Build history of the part. All positions in model axes, mm. Face numbers are marked on the shaded views. A direction names the side the tool comes from. Round coordinates to 2 decimals unless told otherwise and drop trailing zeros. Order: outer loops, then holes, each group sorted by start corner. A loop starts at its lowest first (then second) coordinate and runs counter-clockwise, first axis right, second up. Notation, with made-up numbers: M -31.75,81.5 L 26.25,81.5 A11 ccw 26.25,100.5 Z; hole C 18.25,81.25 d8. An arc over 180 degrees is marked long. One line per item, written item: value. Start each with the question number.
Item 1: Pin check, flat tips, straight feed: pin 1 (3 mm diameter, centred on y = 0.5, z = -3.5, fed in from -X); pin 2 (3 mm diameter, centred on x = -11, y = 1.5, fed in from -Z); pin 3 (2 mm diameter, centred on x = -12, z = 5, fed in from -Y). Stop position of each tip, or through.
Item 2: Tool access for the marked faces 4, 5, 6 and 7: list every direction of +Z, -Z, +X, -X, +Y, -Y with a clear straight run to the whole face (end or side of a thin tool).
Item 3: Band-saw the part on C-C, the plane y = 3.75. Write the cut outline in (x, z).
Item 4: Two-plate mould, pull along Y, no slides. Class the marked faces 1, 2 and 3: +Y half, -Y half, draft (parallel to the pull), parting line (faces both ways), or undercut.
Item 5: Band-saw the part on B-B, the plane z = 2.25. Give the number of separate pieces and of enclosed holes in the cut face, then the cut area to 3 significant figures.
Item 6: Probe L1, parallel to X at y = -3, z = 0.25; L2, parallel to X at y = -1.5, z = 5; L3, parallel to X at y = -4, z = 5.75. List the from-to ranges inside material, lowest first.
Item 7: Band-saw the part on A-A, the plane z = -2.25. Write the cut outline in (x, y), then the cut area to 3 significant figures.
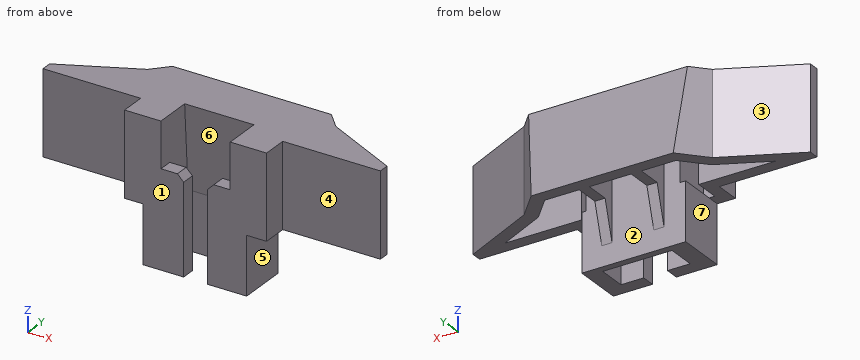
```python
from build123d import *

# Parameters (mm, degrees)
BOSS_EXTRUDE1_DEPTH = 7.4
CUT_EXTRUDE1_DEPTH  = 31.916943618
CHAMFER1_SIZE       = 0.5
CHAMFER1_SIZE_2     = 8
BOSS_EXTRUDE2_DEPTH = 5.1
SKETCH8_W           = 2
SKETCH8_H           = 3.4
BOSS_EXTRUDE5_DEPTH = 1.2
CHAMFER2_SIZE       = 0.55
BOSS_EXTRUDE6_REACH = 19.155
SKETCH9_W           = 0.9
SKETCH9_H           = 3.093590623
SKETCH10_W          = 0.9
SKETCH10_H          = 3.309924143
BOSS_EXTRUDE7_DEPTH = 1
CHAMFER3_SIZE       = 3.5
CHAMFER3_SIZE_2     = 1


with BuildPart() as part:
    # Sketch1 → Boss-Extrude1 (new body)
    with BuildSketch(Plane.XY):
        Polygon((-6.25, 4.137675877), (6.25, 4.137675877), (8.287698915, 1.935907694), (14.849810865, -1.262324123), (14.849810865, -2.162324123), (6.250723489, -2.162324123), (6.25, -4.362324123), (3.05, -4.362324123), (3.05, -1.162324123), (-3.05, -1.162324123), (-3.05, -4.362324123), (-6.25, -4.362324123), (-6.25, -2.162324123), (-14.849810865, -2.162324123), (-14.849810865, -1.262324123), (-8.287698915, 1.935907694), align=None)
    extrude(amount=BOSS_EXTRUDE1_DEPTH)

    # Sketch3 → Cut-Extrude1 (cut, through all)
    with BuildSketch(Plane(origin=(14.849810865, 0, 0), x_dir=(0, 0, -1), z_dir=(1, 0, 0))):
        Polygon((-7.4, 3.337675877), (0, 4.137675877), (-7.4, 4.137675877), align=None)
    extrude(amount=-CUT_EXTRUDE1_DEPTH, mode=Mode.SUBTRACT)

    # Shell1: read off the stored shape, not the designer's step
    # Shell1: loft between two sections, ruled curve by curve
    shell1_from = [
        Edge.make_line((5.15, -1.062324123, 6.3), (11.928689782, -1.062324123, 6.3)),
        Edge.make_line((-11.928689782, -1.062324123, 6.3), (-5.15, -1.062324123, 6.3)),
        Edge.make_line((11.928689782, -1.062324123, 6.3), (7.620430834, 1.037428357, 6.3)),
        Edge.make_line((7.620430834, 1.037428357, 6.3), (6.405496555, 2.350185419, 6.3)),
        Edge.make_line((-6.405496555, 2.350185419, 6.3), (-7.620430834, 1.037428357, 6.3)),
        Edge.make_line((-7.620430834, 1.037428357, 6.3), (-11.928689782, -1.062324123, 6.3)),
        Edge.make_line((-5.15, -1.062324123, 6.3), (-5.15, -3.262324123, 6.3)),
        Edge.make_line((-5.15, -3.262324123, 6.3), (-4.15, -3.262324123, 6.3)),
        Edge.make_line((4.15, -3.262324123, 6.3), (5.15, -3.262324123, 6.3)),
        Edge.make_line((-4.15, -3.262324123, 6.3), (-4.15, -0.062324123, 6.3)),
        Edge.make_line((-4.15, -0.062324123, 6.3), (4.15, -0.062324123, 6.3)),
        Edge.make_line((4.15, -0.062324123, 6.3), (4.15, -3.262324123, 6.3)),
        Edge.make_line((5.15, -3.262324123, 6.3), (5.15, -1.062324123, 6.3)),
        Edge.make_line((6.405496555, 2.350185419, 6.3), (-6.405496555, 2.350185419, 6.3)),
    ]
    shell1_to = [
        Edge.make_line((5.15, -1.062324123, 0), (11.928689782, -1.062324123, 0)),
        Edge.make_line((-11.928689782, -1.062324123, 0), (-5.15, -1.062324123, 0)),
        Edge.make_line((11.928689782, -1.062324123, 0), (7.620430834, 1.037428357, 0)),
        Edge.make_line((7.620430834, 1.037428357, 0), (5.775167626, 3.0312665, 0)),
        Edge.make_line((-5.775167626, 3.0312665, 0), (-7.620430834, 1.037428357, 0)),
        Edge.make_line((-7.620430834, 1.037428357, 0), (-11.928689782, -1.062324123, 0)),
        Edge.make_line((-5.15, -1.062324123, 0), (-5.15, -3.262324123, 0)),
        Edge.make_line((-5.15, -3.262324123, 0), (-4.15, -3.262324123, 0)),
        Edge.make_line((4.15, -3.262324123, 0), (5.15, -3.262324123, 0)),
        Edge.make_line((-4.15, -3.262324123, 0), (-4.15, -0.062324123, 0)),
        Edge.make_line((-4.15, -0.062324123, 0), (4.15, -0.062324123, 0)),
        Edge.make_line((4.15, -0.062324123, 0), (4.15, -3.262324123, 0)),
        Edge.make_line((5.15, -3.262324123, 0), (5.15, -1.062324123, 0)),
        Edge.make_line((5.775167626, 3.0312665, 0), (-5.775167626, 3.0312665, 0)),
    ]
    shell1 = Solid(Shell([*[Face.make_surface_from_curves(shell1_from[k], shell1_to[k]) for k in range(14)], Face(Wire(shell1_from)), Face(Wire(shell1_to))]))
    add(shell1, mode=Mode.SUBTRACT)

    # Chamfer1
    # the kernel refuses this chamfer: 8, 0.5 mm, written as the material it takes off along each edge
    with BuildSketch(Plane(origin=(3.05, -1.162324123, 0), x_dir=(0, 1, 0), z_dir=(-1, 0, 0))) as chamfer1_piece_1:
        Polygon((CHAMFER1_SIZE, 0), (0, -CHAMFER1_SIZE_2), (0, 0), align=None)
    extrude(amount=6.1, mode=Mode.SUBTRACT)

    # Sketch7 → Boss-Extrude2 (add)
    with BuildSketch(Plane(origin=(0, 0, 0), x_dir=(-1, 0, 0), z_dir=(0, 0, -1))):
        Polygon((-3.05, -4.362324123), (-1.05, -4.362324123), (-1.05, -3.162324123), (-3.05, -3.162324123), (-3.05, -0.662324123), (3.05, -0.662324123), (3.05, -3.162324123), (1.05, -3.162324123), (1.05, -4.362324123), (3.05, -4.362324123), (4.65, -4.362324123), (4.65, -0.062324123), (-4.497528609, -0.062324123), (-4.497528609, -4.362324123), align=None)
    extrude(amount=BOSS_EXTRUDE2_DEPTH)

    # Sketch8 → Boss-Extrude5 (add)
    with BuildSketch(Plane(origin=(0, -4.362324123, 0), x_dir=(-1, 0, 0), z_dir=(0, -1, 0))):
        with Locations((-2.05, -1.7)):
            Rectangle(SKETCH8_W, SKETCH8_H)
        with Locations((2.05, -1.7)):
            Rectangle(SKETCH8_W, SKETCH8_H)
    extrude(amount=-BOSS_EXTRUDE5_DEPTH)

    # Chamfer2
    chamfer2_edges = [part.edges().sort_by_distance(p)[0] for p in [
        (1.05, -3.762324123, 3.4),
        (-1.05, -3.762324123, 3.4),
    ]]
    chamfer(chamfer2_edges, length=CHAMFER2_SIZE)

    # Sketch9 → Boss-Extrude6 (add, up to next)
    with BuildSketch(Plane(origin=(0, 0, 0), x_dir=(-1, 0, 0), z_dir=(0, 0, -1)), mode=Mode.PRIVATE) as boss_extrude6_sk1:
        with Locations((-2.288760134, 1.484471189)):
            Rectangle(SKETCH9_W, SKETCH9_H)
    boss_extrude6_tool1 = extrude(boss_extrude6_sk1.sketch, amount=-BOSS_EXTRUDE6_REACH, mode=Mode.PRIVATE) - part.part
    # Sketch9 → Boss-Extrude6 (add, up to next)
    with BuildSketch(Plane(origin=(0, 0, 0), x_dir=(-1, 0, 0), z_dir=(0, 0, -1)), mode=Mode.PRIVATE) as boss_extrude6_sk2:
        with Locations((2.288760134, 1.484471189)):
            Rectangle(SKETCH9_W, SKETCH9_H)
    boss_extrude6_tool2 = extrude(boss_extrude6_sk2.sketch, amount=-BOSS_EXTRUDE6_REACH, mode=Mode.PRIVATE) - part.part
    add(boss_extrude6_tool1.solids().sort_by_distance((2.28876, 1.484471, 0))[0])
    add(boss_extrude6_tool2.solids().sort_by_distance((-2.28876, 1.484471, 0))[0])

    # Sketch10 → Boss-Extrude7 (add)
    with BuildSketch(Plane(origin=(0, -0.062324123, 0), x_dir=(1, 0, 0), z_dir=(0, 1, 0))):
        with Locations((2.288760134, 1.654962072)):
            Rectangle(SKETCH10_W, SKETCH10_H)
        with Locations((-2.288760134, 1.654962072)):
            Rectangle(SKETCH10_W, SKETCH10_H)
    extrude(amount=BOSS_EXTRUDE7_DEPTH)

    # Chamfer3
    # the kernel refuses this chamfer: 3.5, 1 mm, written as the material it takes off along each edge
    with BuildSketch(Plane(origin=(-11.825802237, 0.937675877, -3.309924143), x_dir=(0, 0, 1), z_dir=(1, 0, 0))) as chamfer3_piece_1_section:
        Polygon((CHAMFER3_SIZE, 0), (0, CHAMFER3_SIZE_2), (0, 0), align=None)
    chamfer3_piece_1 = extrude(amount=19.074084206, mode=Mode.PRIVATE)
    chamfer3_piece_1 = split(chamfer3_piece_1, bisect_by=Plane(origin=(-11.825802237, 0.937675877, 0), z_dir=(0, 0, -1)), keep=Keep.TOP, mode=Mode.PRIVATE)
    chamfer3_piece_1 = split(chamfer3_piece_1, bisect_by=Plane(origin=(-11.825802237, -0.062324123, -3.309924143), z_dir=(0, 1, 0)), keep=Keep.TOP, mode=Mode.PRIVATE)
    add(chamfer3_piece_1, mode=Mode.SUBTRACT)
    with BuildSketch(Plane(origin=(-7.248281969, 0.937675877, -3.309924143), x_dir=(0, 0, 1), z_dir=(1, 0, 0))) as chamfer3_piece_2_section:
        Polygon((CHAMFER3_SIZE, 0), (0, CHAMFER3_SIZE_2), (0, 0), align=None)
    chamfer3_piece_2 = extrude(amount=19.074084206, mode=Mode.PRIVATE)
    chamfer3_piece_2 = split(chamfer3_piece_2, bisect_by=Plane(origin=(-7.248281969, 0.937675877, 0), z_dir=(0, 0, -1)), keep=Keep.TOP, mode=Mode.PRIVATE)
    chamfer3_piece_2 = split(chamfer3_piece_2, bisect_by=Plane(origin=(-7.248281969, -0.062324123, -3.309924143), z_dir=(0, 1, 0)), keep=Keep.TOP, mode=Mode.PRIVATE)
    add(chamfer3_piece_2, mode=Mode.SUBTRACT)


solid = part.part
```
Output:
1. pin 1: stops at x = -4.65
1. pin 2: stops at z = 0
1. pin 3: stops at y = -2.16
2. face 4: +Z, -Z, +X, -Y
2. face 5: -Z, +X, +Y, -Y
2. face 6: -Z
2. face 7: -Z, -X, +Y, -Y
3. outline: M -6.61,0 L 6.61,0 L 6.61,3.59 L -6.61,3.59 Z
4. face 1: -Y half
4. face 2: undercut
4. face 3: +Y half
5. separate pieces: 1
5. enclosed holes: 3
5. area: 84.4 mm²
6. L1: x = -6.25 to -5.15, -4.15 to -3.05, 3.05 to 4.15, 5.15 to 6.25
6. L2: x = -14.85 to -5.15, -4.15 to -3.05, 3.05 to 4.15, 5.15 to 14.85
6. L3: x = -6.25 to -3.05, 3.05 to 6.25
7. outline: M -4.65,-4.36 L -1.05,-4.36 L -1.05,-3.16 L -3.05,-3.16 L -3.05,-0.66 L 3.05,-0.66 L 3.05,-3.16 L 1.05,-3.16 L 1.05,-4.36 L 4.5,-4.36 L 4.5,-0.06 L 2.74,-0.06 L 2.74,0.24 L 1.84,0.24 L 1.84,-0.06 L -1.84,-0.06 L -1.84,0.24 L -2.74,0.24 L -2.74,-0.06 L -4.65,-0.06 Z
7. area: 22.1 mm²
